The listing builds one solid part. Answer for the finished solid, in the listing's coordinates (mm). Coordinates: 2 decimals unless noted, no trailing zeros. Order: outer loops, then holes, each group sorted by start corner. A loop starts at its lowest first (then second) coordinate and runs counter-clockwise, first axis right, second up. Notation, with made-up numbers: (46.5, 52) -> (88.5, 52) arc R20 ccw to (88.5, 91) -> close; hole circle Ø6 at (-20, 20.25). An arc over 180 degrees is marked (long way). Answer in a Markdown table with one row per item.
```python
from build123d import *

# Parameters (mm, degrees)
SKETCH1_R           = 35
BOSS_EXTRUDE1_DEPTH = 5
SKETCH2_R           = 3.1
CUT_EXTRUDE1_DEPTH  = 50.749371855
SKETCH5_R           = 35
CUT_EXTRUDE4_DEPTH  = 2


with BuildPart() as part:
    # Sketch1 → Boss-Extrude1 (new body)
    with BuildSketch(Plane(origin=(0, 0, 0), x_dir=(1, 0, 0), z_dir=(0, 1, 0))):
        with Locations(Location((0, 0, 0), (0, 0, 270))):
            Circle(SKETCH1_R)
    extrude(amount=BOSS_EXTRUDE1_DEPTH)

    # Sketch2 → Cut-Extrude1 (cut, through all)
    with BuildSketch(Plane(origin=(0, 5, 0), x_dir=(1, 0, 0), z_dir=(0, 1, 0))):
        with Locations(Location((-17.67766953, 17.67766953, 0), (0, 0, 270))):
            Circle(SKETCH2_R)
        with Locations(Location((17.67766953, 17.67766953, 0), (0, 0, 270))):
            Circle(SKETCH2_R)
        with Locations(Location((17.67766953, -17.67766953, 0), (0, 0, 270))):
            Circle(SKETCH2_R)
        with Locations(Location((-17.67766953, -17.67766953, 0), (0, 0, 270))):
            Circle(SKETCH2_R)
    extrude(amount=-CUT_EXTRUDE1_DEPTH, mode=Mode.SUBTRACT)

    # Sketch5 → Cut-Extrude4 (cut)
    with BuildSketch(Plane.XZ):
        with Locations(Location((0, 0, 0), (0, 0, 90))):
            Circle(SKETCH5_R)
    extrude(amount=-CUT_EXTRUDE4_DEPTH, mode=Mode.SUBTRACT)


solid = part.part
```
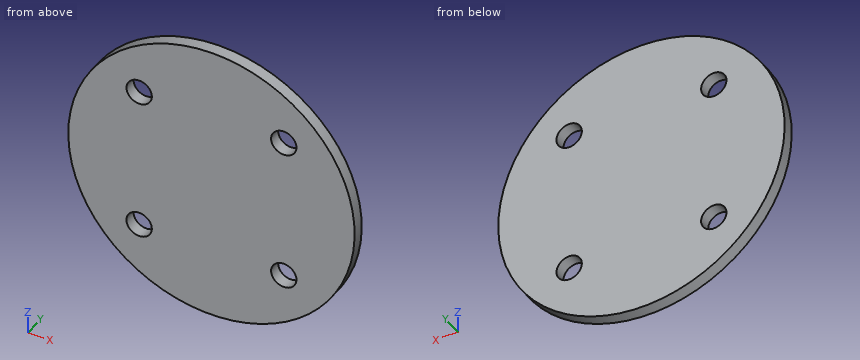
(1) A cutting plane is placed at A-A, the plane z = 16. Determine the outline of the cut face in (x, y), then the cut area to 3 significant figures.
Check values:
| item | result |
|---|---|
| outline | (-31.13, 2) -> (-20.28, 2) -> (-20.28, 5) -> (-31.13, 5) -> close; (-15.07, 2) -> (15.07, 2) -> (15.07, 5) -> (-15.07, 5) -> close; (20.28, 2) -> (31.13, 2) -> (31.13, 5) -> (20.28, 5) -> close |
| area | 155 mm² |
(2) A cutting plane is placed at B-B, the plane y = 4.2. Determine the outline of the cut face in (x, z).
Check values:
| item | result |
|---|---|
| outline | circle Ø70 at (0, 0); hole circle Ø6.2 at (-17.68, -17.68); hole circle Ø6.2 at (-17.68, 17.68); hole circle Ø6.2 at (17.68, -17.68); hole circle Ø6.2 at (17.68, 17.68) |
(3) A cutting plane is placed at D-D, the plane x = -6.5. Determine the outline of the cut face in (y, z).
Check values:
| item | result |
|---|---|
| outline | (2, -34.39) -> (5, -34.39) -> (5, 34.39) -> (2, 34.39) -> close |
(4) Flat-ended cylindrical pins translate along their axes: pin 1 (5.5 mm diameter, centred on x = -17.68, z = -17.68, fed in from +Y); pin 2 (1.5 mm diameter, centred on y = 4, z = 25.5, fed in from +X); pin 3 (1 mm diameter, centred on x = 13, y = 3, fed in from +Z). Find the tip coordinate at first contact, or state that the pin passes through.
Check values:
| item | result |
|---|---|
| pin 1 | through |
| pin 2 | x = 24.75 |
| pin 3 | z = 32.69 |
(5) A cutting plane is placed at C-C, the plane z = -19.5. Determine the outline of the cut face in (x, y).
Check values:
| item | result |
|---|---|
| outline | (-29.06, 2) -> (-20.19, 2) -> (-20.19, 5) -> (-29.06, 5) -> close; (-15.17, 2) -> (15.17, 2) -> (15.17, 5) -> (-15.17, 5) -> close; (20.19, 2) -> (29.06, 2) -> (29.06, 5) -> (20.19, 5) -> close |
(6) Find the intervals of material crossed by line 1 along Z through (x, y) = (-19, 3.95); line 2 along X through (y, z) = (4, 15); line 3 along Z through (x, y) = (15.5, 2.4), in increasing order. Write a range as from..to.
Check values:
| item | result |
|---|---|
| line 1 | -29.39..-20.48, -14.87..14.87, 20.48..29.39 |
| line 2 | -31.62..-19.24, -16.12..16.12, 19.24..31.62 |
| line 3 | -31.38..-19.88, -15.47..15.47, 19.88..31.38 |
